```python
from build123d import *

# Parameters (mm, degrees)
BOSS_EXTRUDE1_DEPTH   = 1.5875
FILLET1_R             = 9.525
F_8_CLEARANCE_HOLE1_D = 4.4958


with BuildPart() as part:
    # Sketch2 → Boss-Extrude1 (new, symmetric)
    with BuildSketch(Plane.XY):
        Polygon((37.010512242, 0), (69.85, 32.839487758), (69.85, 69.85), (44.45, 69.85), (44.45, 47.850640303), (21.999359697, 25.4), (0, 25.4), (0, 0), align=None)
    extrude(amount=BOSS_EXTRUDE1_DEPTH, both=True)

    # Fillet1
    fillet1_edges = [part.edges().sort_by_distance(p)[0] for p in [
        (69.85, 32.839487758, 0),
        (37.010512242, 0, 0),
        (0, 0, 0),
        (0, 25.4, 0),
        (21.999359697, 25.4, 0),
        (44.45, 47.850640303, 0),
        (44.45, 69.85, 0),
        (69.85, 69.85, 0),
    ]]
    fillet(fillet1_edges, radius=FILLET1_R)

    # #8 Clearance Hole1 (through all)
    with Locations(Plane.XY.offset(1.5875)):
        with Locations((12.7, 12.7), (31.75, 12.7), (57.15, 38.1), (57.15, 57.15)):
            Hole(F_8_CLEARANCE_HOLE1_D / 2)


solid = part.part
```
Geometry: final body of the model. Coordinates: model frame, mm. A direction names the side the tool comes from. Coordinates: 2 decimals unless noted, no trailing zeros. Order: outer loops, then holes, each group sorted by start corner. A loop starts at its lowest first (then second) coordinate and runs counter-clockwise, first axis right, second up. Notation, with made-up numbers: (-34, 47) -> (6, 47) arc R20 cw to (6, 67) -> close; hole circle Ø11 at (75, 85.5). An arc over 180 degrees is marked (long way). Use CSV: the item, a comma, the result in double quotes.
1) Pin query (flat end, axial travel): pin 1 Ø1.5 at (x, z) = (37, -1) entering from -Y; pin 2 Ø1.6 at (x, z) = (13, 0.5) entering from +Y; pin 3 Ø4 at (x, y) = (42.5, 62) entering from -Z. Return the tip coordinate at first contact, or that it passes through.
Findings:
pin 1,"stops at y = 0.55"
pin 2,"stops at y = 25.4"
pin 3,"passes through"
2) Section D-D on x = 57.15. Output: boundary loops of the cut face in (y, z), then the cut area to 3 significant figures.
Findings:
outline,"(20.14, -1.59) -> (35.85, -1.59) -> (35.85, 1.59) -> (20.14, 1.59) -> close; (40.35, -1.59) -> (54.9, -1.59) -> (54.9, 1.59) -> (40.35, 1.59) -> close; (59.4, -1.59) -> (69.85, -1.59) -> (69.85, 1.59) -> (59.4, 1.59) -> close"
area,"129 mm^2"
3) Line query: line 1 (Y direction, x = 12.7, z = -0.1); line 2 (Y direction, x = 57.15, z = 0.7); line 3 (X direction, y = 14.5, z = 0.1). Output: solid intervals per line, ascending.
Findings:
line 1,"y = 0 to 10.45, 14.95 to 25.4"
line 2,"y = 20.14 to 35.85, 40.35 to 54.9, 59.4 to 69.85"
line 3,"x = 0 to 11.35, 14.05 to 30.4, 33.1 to 51.51"
4) Section A-A on z = -0.65. Output: boundary loops of the cut face in (x, y) (3 decimals), then the cut area to 3 significant figures.
Findings:
outline,"(0, 9.525) arc R9.525 ccw to (9.525, 0) -> (33.065, 0) arc R9.525 ccw to (39.8, 2.79) -> (67.06, 30.05) arc R9.525 ccw to (69.85, 36.785) -> (69.85, 60.325) arc R9.525 ccw to (60.325, 69.85) -> (53.975, 69.85) arc R9.525 ccw to (44.45, 60.325) -> (44.45, 51.796) arc R9.525 cw to (41.66, 45.061) -> (24.789, 28.19) arc R9.525 cw to (18.054, 25.4) -> (9.525, 25.4) arc R9.525 ccw to (0, 15.875) -> close; hole circle Ø4.496 at (12.7, 12.7); hole circle Ø4.496 at (31.75, 12.7); hole circle Ø4.496 at (57.15, 38.1); hole circle Ø4.496 at (57.15, 57.15)"
area,"2,470 mm^2"
5) Section C-C on x = 12.7. Output: boundary loops of the cut face in (y, z), then the cut area to 3 significant figures.
Findings:
outline,"(0, -1.59) -> (10.45, -1.59) -> (10.45, 1.59) -> (0, 1.59) -> close; (14.95, -1.59) -> (25.4, -1.59) -> (25.4, 1.59) -> (14.95, 1.59) -> close"
area,"66.4 mm^2"
6) Section B-B on y = 57.15. Output: boundary loops of the cut face in (x, z).
Findings:
outline,"(44.45, -1.59) -> (54.9, -1.59) -> (54.9, 1.59) -> (44.45, 1.59) -> close; (59.4, -1.59) -> (69.85, -1.59) -> (69.85, 1.59) -> (59.4, 1.59) -> close"
7) Mould query, pull axis X, two halves, no side actions, for faces 1 (the flat face through (21, 0, 0)), 2 (the cylindrical face through (58.807, 58.669, -0.022)), 3 (the flat face through (44.45, 56, 0)). Classes: +X half, -X half, draft (parallel to the pull), parting line (faces both ways), or undercut.
Findings:
face 1,"draft"
face 2,"undercut"
face 3,"-X half"
8) Access query for faces 4 (the flat face through (42, 28, 1.588)), 5 (the flat face through (14, 25.4, 0)). Directions: +Z, -Z, +X, -X, +Y, -Y. A direction counts if a zero-diameter tool reaches every point of the face in a straight line with its end or side. Return the directions, or none.
Findings:
face 4,"+Z, +X, -X, +Y, -Y"
face 5,"+Z, -Z, -X, +Y"
